from build123d import *

# Parameters (mm, degrees)
F0_W      = 71.12
F0_H      = 2.54
F1_DEPTH  = 22.86
F2_W      = 68.58
F2_H      = 1.27
F3_DEPTH  = 22.86
F4_W      = 0.762
F4_H      = 22.352
F5_DEPTH  = 1.905
F6_W      = 0.762
F6_H      = 22.352
F7_DEPTH  = 1.905
F8_R      = 0.127
F9_DEPTH  = 0.762
F10_R     = 0.127
F11_DEPTH = 0.762
F12_W     = 5.08
F12_H     = 0.762
F13_DEPTH = 2.54
F14_W     = 4.064
F14_H     = 2.032
F15_DEPTH = 2.287
F16_W     = 4.064
F16_H     = 2.032
F17_DEPTH = 2.287
F18_W     = 0.635
F18_H     = 0.635
F19_DEPTH = 0.635
F20_R     = 0.1905
F21_DEPTH = 2.54


with BuildPart() as f1:
    # F0 (on Front) → F1 (new body)
    with BuildSketch(Plane.XZ):
        with Locations((12.489298, 22.094047)):
            Rectangle(F0_W, F0_H)
    extrude(amount=F1_DEPTH)

    # F2 (on face) → F3 (cut)
    with BuildSketch(Plane.XZ.offset(22.86)):
        with Locations((12.489298, 21.459047)):
            Rectangle(F2_W, F2_H)
    extrude(amount=-F3_DEPTH, mode=Mode.SUBTRACT)

    # F4 (on face) → F5 (cut)
    with BuildSketch(Plane(origin=(0, 0, 20.824047), x_dir=(1, 0, 0), z_dir=(0, 0, -1))):
        with Locations((47.414298, 11.43)):
            Rectangle(F4_W, F4_H)
    extrude(amount=-F5_DEPTH, mode=Mode.SUBTRACT)

    # F6 (on face) → F7 (cut)
    with BuildSketch(Plane(origin=(0, 0, 20.824047), x_dir=(1, 0, 0), z_dir=(0, 0, -1))):
        with Locations((-22.435702, 11.43)):
            Rectangle(F6_W, F6_H)
    extrude(amount=-F7_DEPTH, mode=Mode.SUBTRACT)

    # F8 (on face) → F9 (join, through all)
    with BuildSketch(Plane(origin=(47.795298, 0, 0), x_dir=(0, -1, 0), z_dir=(-1, 0, 0))):
        with Locations((16.51, 21.459047)):
            Circle(F8_R)
        with Locations((6.35, 21.586047)):
            Circle(F8_R)
    extrude(amount=F9_DEPTH)

    # F10 (on face) → F11 (join, through all)
    with BuildSketch(Plane(origin=(-22.054702, 0, 0), x_dir=(0, -1, 0), z_dir=(-1, 0, 0))):
        with Locations((16.51, 21.459047)):
            Circle(F10_R)
        with Locations((6.35, 21.459047)):
            Circle(F10_R)
    extrude(amount=F11_DEPTH)

    # F12 (on face) → F13 (join)
    with BuildSketch(Plane.XZ.offset(22.86)):
        with Locations((-0.210702, 22.729047)):
            Rectangle(F12_W, F12_H)
        with Locations((25.189298, 22.729047)):
            Rectangle(F12_W, F12_H)
    extrude(amount=F13_DEPTH)

    # F14 (on face) → F15 (cut, through all)
    with BuildSketch(Plane.XY.offset(23.110047)):
        with Locations((25.189298, -23.876)):
            Rectangle(F14_W, F14_H)
    extrude(amount=-F15_DEPTH, mode=Mode.SUBTRACT)

    # F16 (on face) → F17 (cut, through all)
    with BuildSketch(Plane.XY.offset(23.110047)):
        with Locations((-0.210702, -23.876)):
            Rectangle(F16_W, F16_H)
    extrude(amount=-F17_DEPTH, mode=Mode.SUBTRACT)

    # F18 (on face) → F19 (join)
    with BuildSketch(Plane.XZ.offset(22.86)):
        with Locations((45.436141, 23.046547)):
            Rectangle(F18_W, F18_H)
        with Locations((44.179277, 22.411547)):
            Rectangle(F18_W, F18_H)
        with Locations((41.867119, 22.411547)):
            Rectangle(F18_W, F18_H)
    extrude(amount=F19_DEPTH)

    # F20 (on face) → F21 (cut)
    with BuildSketch(Plane.YZ.offset(45.753641)):
        with Locations((-23.1775, 23.063494)):
            Circle(F20_R)
    extrude(amount=-F21_DEPTH, mode=Mode.SUBTRACT)


solid = f1.part
Could you check a few things on this model? Use its own coordinates, in mm. A direction names the side the tool comes from. Coordinates: 2 decimals unless noted, no trailing zeros. Write each loop counter-clockwise with the first axis right and the second up, starting at its lowest first coordinate (ties: lowest second). Pieces come first, ordered by that corner, then holes. Notation, with made-up numbers: M 26,36.5 L 79,36.5 A11 cw 79,41.5 Z; hole C 6.25,-25.75 d1. An arc over 180 degrees is marked long. One line per question, with ' | ' between items.
1) Imagine slicing it at B-B, the plane x = 5.5. Write out the boundary of the cut face in (y, z).
Checks:
outline: M -22.86,22.09 L 0,22.09 L 0,23.36 L -22.86,23.36 Z
2) For pin 1 Ø5 at (x, y) = (-7, -6.5) entering from -Z; pin 2 Ø0.6 at (y, z) = (-24, 22.5) entering from -X; pin 3 Ø0.8 at (y, z) = (-24.5, 22.5) entering from +X, each with a flat end and sliding along its axis, tell me the tip position at first contact or that it passes through.
Checks:
pin 1: z = 22.09 | pin 2: x = -2.75 | pin 3: x = 27.73
3) If we mould it in two halves opening along Y, with no side actions, what happens to faces 1 (the face through (47.795, -11, 22)), 2 (the face through (12, 0, 23)), 3 (the face through (25.2, -25.2, 23.11)), 4 (the face through (47.033, -11, 22))? For each: released by +Y, released by -Y, zero draft, split by the parting line, or undercut.
Checks:
face 1: undercut | face 2: released by +Y | face 3: zero draft | face 4: undercut
4) I need wall thicknesses on probe 1 along X at (y, z) = (-11.5, 21.7); probe 2 along X at (y, z) = (-23.75, 22.9); probe 3 along X at (y, z) = (-14.75, 22.3). Which ranges of each line are inside material? Lowest first, please. Write a range as [from, to].
Checks:
probe 1: [-23.07, -22.82], [-22.05, -21.8], [46.78, 47.03], [47.8, 48.05] | probe 2: [-2.75, -2.24], [1.82, 2.33], [22.65, 23.16], [27.22, 27.73] | probe 3: [-23.07, -22.82], [-22.05, 47.03], [47.8, 48.05]
5) Imagine slicing it at A-A, the plane y = -20. Write out the boundary of the cut face in (x, z), and give its area (3 significant figures).
Checks:
outline: M -23.07,20.82 L -22.82,20.82 L -22.82,22.73 L -22.05,22.73 L -22.05,20.82 L -21.8,20.82 L -21.8,22.09 L 46.78,22.09 L 46.78,20.82 L 47.03,20.82 L 47.03,22.73 L 47.8,22.73 L 47.8,20.82 L 48.05,20.82 L 48.05,23.36 L -23.07,23.36 Z | area: 90.6 mm²
6) For faces 5 (the face through (-21.801, -12, 21)), 6 (the face through (-23.071, -11, 22)), 7 (the face through (25.2, -25.2, 22.348)), which set-ups out of +Z, -Z, +X, -X, +Y, -Y let a thin tool reach every point of the face, with its end or its side?
Checks:
face 5: -Z, +Y, -Y | face 6: +Z, -Z, -X, +Y, -Y | face 7: -Z, -X, -Y
